```python
from build123d import *

# Parameters (mm, degrees)
CUT_EXTRUDE_START   = 10
CUT_EXTRUDE_1_DEPTH = 2.5
SKETCH_4_W          = 1.2
SKETCH_4_H          = 1
EXTRUDE_START       = -99.8
EXTRUDE_11_DEPTH    = 35.8
CHAMFER_1_SIZE      = 2


with BuildPart() as part:
    # 草图1 → 旋转1 (revolve)
    with BuildSketch(Plane.XY, mode=Mode.PRIVATE) as revolve_1_sk:
        with BuildLine():
            Line((0, 10), (0, 0))
            Line((0, 0), (226, 0))
            Line((226, 0), (226, 10))
            Line((226, 10), (162, 10))
            Line((162, 10), (162, 12.5))
            Line((162, 12.5), (97.723805295, 12.5))
            ThreePointArc((97.723805295, 12.5), (91.807725512, 13.81142246), (87, 17.5))
            Line((87, 17.5), (72, 17.5))
            Line((72, 17.5), (72, 12.5))
            Line((72, 12.5), (45, 12.5))
            Line((45, 12.5), (45, 10))
            Line((45, 10), (0, 10))
        make_face()
    revolve(revolve_1_sk.sketch.rotate(Axis((0, 0, 0), (1, 0, 0)), 90), axis=Axis((0, 0, 0), (1, 0, 0)))

    # 草图3 → 切除-拉伸1 (cut)
    with BuildSketch(Plane(origin=(0, 0, 0), x_dir=(1, 0, 0), z_dir=(0, 1, 0)).offset(CUT_EXTRUDE_START)):
        with BuildLine():
            Line((-33, 3), (33, 3))
            ThreePointArc((33, 3), (36, 0), (33, -3))
            Line((33, -3), (-33, -3))
            ThreePointArc((-33, -3), (-36, 0), (-33, 3))
        make_face()
    extrude(amount=-CUT_EXTRUDE_1_DEPTH, mode=Mode.SUBTRACT)

    # 草图4 → 切除-旋转1 (revolve, cut)
    with BuildSketch(Plane.XY, mode=Mode.PRIVATE) as cut_revolve_1_sk:
        with Locations((54.4, 12)):
            Rectangle(SKETCH_4_W, SKETCH_4_H)
        with Locations((54.4, -12)):
            Rectangle(SKETCH_4_W, SKETCH_4_H)
    revolve(cut_revolve_1_sk.sketch.rotate(Axis((0, 0, 0), (1, 0, 0)), 90), axis=Axis((0, 0, 0), (1, 0, 0)), mode=Mode.SUBTRACT)

    # 草图5 → 切除-旋转2 (revolve, cut)
    with BuildSketch(Plane.XY, mode=Mode.PRIVATE) as cut_revolve_2_sk:
        with BuildLine():
            Line((162, 12.5), (126.2, 12.5))
            ThreePointArc((126.2, 12.5), (131.507077415, 10.633014138), (137.097247359, 10))
            Line((137.097247359, 10), (162, 10))
            Line((162, 10), (162, 12.5))
        make_face()
    revolve(cut_revolve_2_sk.sketch.rotate(Axis((0, 0, 0), (1, 0, 0)), 90), axis=Axis((0, 0, 0), (1, 0, 0)), mode=Mode.SUBTRACT)

    # 草图8 → 凸台-拉伸11 (add)
    with BuildSketch(Plane(origin=(226, 0, 0), x_dir=(0, 0, -1), z_dir=(1, 0, 0)).offset(EXTRUDE_START)):
        with BuildLine():
            Line((9.356601718, 8.288787866), (7.581760866, 7.264083023))
            ThreePointArc((7.581760866, 7.264083023), (5.25, 9.09326674), (2.5, 10.198039027))
            Line((2.5, 10.198039027), (2.5, 12.247448714))
            ThreePointArc((2.5, 12.247448714), (0, 12.5), (-2.5, 12.247448714))
            Line((-2.5, 12.247448714), (-2.5, 10.198039027))
            ThreePointArc((-2.5, 10.198039027), (-5.25, 9.09326674), (-7.581760866, 7.264083023))
            Line((-7.581760866, 7.264083023), (-9.356601718, 8.288787866))
            ThreePointArc((-9.356601718, 8.288787866), (-10.825317547, 6.25), (-11.856601718, 3.958660847))
            Line((-11.856601718, 3.958660847), (-10.081760866, 2.933956004))
            ThreePointArc((-10.081760866, 2.933956004), (-10.5, 0), (-10.081760866, -2.933956004))
            Line((-10.081760866, -2.933956004), (-11.856601718, -3.958660847))
            ThreePointArc((-11.856601718, -3.958660847), (-10.825317547, -6.25), (-9.356601718, -8.288787866))
            Line((-9.356601718, -8.288787866), (-7.581760866, -7.264083023))
            ThreePointArc((-7.581760866, -7.264083023), (-5.25, -9.09326674), (-2.5, -10.198039027))
            Line((-2.5, -10.198039027), (-2.5, -12.247448714))
            ThreePointArc((-2.5, -12.247448714), (0, -12.5), (2.5, -12.247448714))
            Line((2.5, -12.247448714), (2.5, -10.198039027))
            ThreePointArc((2.5, -10.198039027), (5.25, -9.09326674), (7.581760866, -7.264083023))
            Line((7.581760866, -7.264083023), (9.356601718, -8.288787866))
            ThreePointArc((9.356601718, -8.288787866), (10.825317547, -6.25), (11.856601718, -3.958660847))
            Line((11.856601718, -3.958660847), (10.081760866, -2.933956004))
            ThreePointArc((10.081760866, -2.933956004), (10.5, 0), (10.081760866, 2.933956004))
            Line((10.081760866, 2.933956004), (11.856601718, 3.958660847))
            ThreePointArc((11.856601718, 3.958660847), (10.825317547, 6.25), (9.356601718, 8.288787866))
        make_face()
    extrude(amount=EXTRUDE_11_DEPTH)

    # 倒角1
    chamfer_1_edges = [part.edges().sort_by_distance(p)[0] for p in [
        (226, 0, -10),
        (162, 6.25, -10.825317547),
        (162, -6.25, -10.825317547),
        (162, -12.5, 0),
        (162, -6.25, 10.825317547),
        (162, 6.25, 10.825317547),
        (162, 12.5, 0),
        (72, 0, -17.5),
        (45, 0, -12.5),
        (0, -8.062257748, -5.916079783),
    ]]
    chamfer(chamfer_1_edges, length=CHAMFER_1_SIZE)


solid = part.part
```
Can you work these out from the model? Positions are in its coordinate system, mm. A direction names the side the tool comes from. Give positions to 0.01 mm unless a question says otherwise; leave off trailing zeros. Write each loop counter-clockwise with the first axis right and the second up, starting at its lowest first coordinate (ties: lowest second). Pieces come first, ordered by that corner, then holes. Notation, with made-up numbers: (48, 20) -> (97, 20) arc R15 cw to (97, 36) -> close; hole circle Ø5 at (72.5, 39). An arc over 180 degrees is marked (long way). Write item = value, one per line.
(1) Suppose I cut it at A-A on x = 157. Write out the boundary of the cut face in (y, z).
Worked out:
outline = (-12.25, -2.5) -> (-10.2, -2.5) arc R10.5 ccw to (-7.26, -7.58) -> (-8.29, -9.36) arc R12.5 ccw to (-3.96, -11.86) -> (-2.93, -10.08) arc R10.5 ccw to (2.93, -10.08) -> (3.96, -11.86) arc R12.5 ccw to (8.29, -9.36) -> (7.26, -7.58) arc R10.5 ccw to (10.2, -2.5) -> (12.25, -2.5) arc R12.5 ccw to (12.25, 2.5) -> (10.2, 2.5) arc R10.5 ccw to (7.26, 7.58) -> (8.29, 9.36) arc R12.5 ccw to (3.96, 11.86) -> (2.93, 10.08) arc R10.5 ccw to (-2.93, 10.08) -> (-3.96, 11.86) arc R12.5 ccw to (-8.29, 9.36) -> (-7.26, 7.58) arc R10.5 ccw to (-10.2, 2.5) -> (-12.25, 2.5) arc R12.5 ccw to start
(2) I need wall thicknesses on probe 1 along Z at (x, y) = (158, 8); probe 2 along Y at (x, z) = (205.5, 0.5); probe 3 along X at (y, z) = (0.5, -8). Which ranges of each line are inside material? Lowest first, please. Write a range as from..to.
Worked out:
probe_1 = -9.6..-8.86, -6.8..6.8, 8.86..9.6
probe_2 = -9.99..9.99
probe_3 = 0.02..225.98
(3) Suppose I cut it at C-C on x = 203. Write out the boundary of the cut face in (y, z).
Worked out:
outline = circle Ø20 at (0, 0)
(4) For faces 1 (the face through (193, 0, -10)), 2 (the face through (146.85, 9.07, -5.29)), 3 (the face through (54.4, -11.4, -1.5)), which set-ups out of +Z, -Z, +X, -X, +Y, -Y let a thin tool reach every point of the face, with its end or its side?
Worked out:
face_1 = +X
face_2 = +X, +Y
face_3 = none
(5) Suppose I cut it at B-B on x = 70. Write out the boundary of the cut face in (y, z).
Worked out:
outline = circle Ø25 at (0, 0)
(6) Thinking about a two-plate mould opening in Y: for faces 4 (the face through (55, 4, -11)), 5 (the face through (80.409, 17.084, -3.794)), 6 (the face through (146.9, 0, -10.5)), which applies, released by +Y, released by -Y, zero draft, split by the parting line, or undercut?
Worked out:
face_4 = zero draft
face_5 = split by the parting line
face_6 = undercut
(7) I'm going to push flat-ended pins straight in: P1, Ø0.6, axis at x = 142, y = 11, coming from the +Z side; P2, Ø2, axis at y = 12.5, z = -8.5, coming from the -X side; P3, Ø10, axis at x = 175, y = 14, coming from the -Z side. Where does each tip first touch, or does it pass through?
Worked out:
P1 = 2.5
P2 = 72
P3 = -4.36
